Can you work these out from the model? Positions are in its coordinate system, mm. Face numbers are marked on the shaded views. A direction names the side the tool comes from. Give positions to 0.01 mm unless a question says otherwise; leave off trailing zeros. Loops run counter-clockwise (first coordinate to the right, second up) from the corner with the lowest first, then second, coordinate; pieces in that order, holes last.
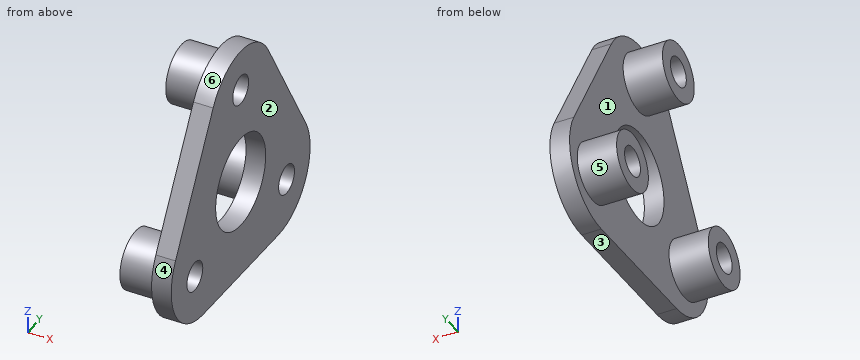
from build123d import *

# Parameters (mm, degrees)
SKETCH_R      = 4.725
SKETCH_R_2    = 1.5
PAD_DEPTH     = 2
SKETCH001_R   = 3
SKETCH001_R_2 = 1.5
PAD001_DEPTH  = 4
FILLET_R      = 6


with BuildPart() as part:
    # Sketch → Pad (new body)
    with BuildSketch(Plane.YZ):
        Polygon((0, 20.207259), (-17.5, -10.10363), (17.5, -10.10363), align=None)
        Circle(SKETCH_R, mode=Mode.SUBTRACT)
        with Locations((0, 10)):
            Circle(SKETCH_R_2, mode=Mode.SUBTRACT)
        with Locations((-8.660254, -5)):
            Circle(SKETCH_R_2, mode=Mode.SUBTRACT)
        with Locations((8.660254, -5)):
            Circle(SKETCH_R_2, mode=Mode.SUBTRACT)
    extrude(amount=-PAD_DEPTH)

    # Sketch001 (on Face9 of Pad) → Pad001 (join)
    with BuildSketch(Plane(origin=(-2, 0, 0), x_dir=(0, 1, 0), z_dir=(-1, 0, 0))):
        with Locations((8.660254, 5)):
            Circle(SKETCH001_R)
        with Locations((8.660254, 5)):
            Circle(SKETCH001_R_2, mode=Mode.SUBTRACT)
        with Locations((-8.660254, 5)):
            Circle(SKETCH001_R)
        with Locations((-8.660254, 5)):
            Circle(SKETCH001_R_2, mode=Mode.SUBTRACT)
        with Locations((0, -10)):
            Circle(SKETCH001_R)
        with Locations((0, -10)):
            Circle(SKETCH001_R_2, mode=Mode.SUBTRACT)
    extrude(amount=PAD001_DEPTH)

    # Fillet
    fillet_edges = [part.edges().sort_by_distance(p)[0] for p in [
        (-1, 0, 20.207259),
        (-1, -17.5, -10.10363),
        (-1, 17.5, -10.10363),
    ]]
    fillet(fillet_edges, radius=FILLET_R)


solid = part.part
(1) Suppose I cut it at C-C on z = 0. List the corners of the cut face in (x, y) for me (3 decimals).
Returned:
outline: (-2, -11.667) - (0, -11.667) - (0, -4.725) - (-2, -4.725) - close; (-2, 4.725) - (0, 4.725) - (0, 11.667) - (-2, 11.667) - close
(2) Please list where these lines run through material, in increasing order: probe 1 along Z at (x, y) = (-0.6, 0) (3 decimals); probe 2 along Y at (x, z) = (-4.2, 10); probe 3 along Y at (x, z) = (-0.4, -5.5).
Returned:
probe 1: z = -10.104 to -4.725, 4.725 to 8.5, 11.5 to 14.207
probe 2: y = -3 to -1.5, 1.5 to 3
probe 3: y = -12.94 to -10.07, -7.25 to 7.25, 10.07 to 12.94
(3) Which directions (+Z, -Z, +X, -X, +Y, -Y) give clear straight access to the entire face, cutting with the end or side of a thin tool? Please do the marked faces 1 and 2.
Returned:
face 1: -X
face 2: +Z, -Z, +X, +Y, -Y
(4) Will these pins go through, and if not, where does the flat tip stop? P1, Ø8, axis at y = 8, z = 3, coming from the +X side; P2, Ø2, axis at x = -1, y = 3.5, coming from the +Z side; P3, Ø1.5, axis at x = -3, y = 3.5, coming from the +Z side; P4, Ø3, axis at x = -2, z = 6, coming from the -Y side.
Returned:
P1: stops at x = 0
P2: stops at z = 13.66
P3: stops at z = 11.2
P4: stops at y = -9.07
(5) Suppose I cut it at A-A on x = -4.2. List the corners of the cut face in (y, z) for me, plus the area to 3 significant figures.
Returned:
outline: circle Ø6 at (-8.66, -5); circle Ø6 at (0, 10); circle Ø6 at (8.66, -5); hole circle Ø3 at (-8.66, -5); hole circle Ø3 at (0, 10); hole circle Ø3 at (8.66, -5)
area: 63.6 mm2
(6) Suppose I cut it at B-B on y = 0. List the corners of the cut face in (x, z) for me (3 decimals), plus the area to 3 significant figures.
Returned:
outline: (-6, 7) - (-2, 7) - (-2, 4.725) - (0, 4.725) - (0, 8.5) - (-6, 8.5) - close; (-6, 11.5) - (0, 11.5) - (0, 14.207) - (-2, 14.207) - (-2, 13) - (-6, 13) - close; (-2, -10.104) - (0, -10.104) - (0, -4.725) - (-2, -4.725) - close
area: 35.7 mm2
(7) Thinking about a two-plate mould opening in Y: for the marked faces 3, 4, 5 and 6, which applies, pulls with the +Y half, pulls with the -Y half, needs draft (parallel to the pull), parting line crosses it, or undercut?
Returned:
face 3: needs draft
face 4: pulls with the -Y half
face 5: undercut
face 6: parting line crosses it
(8) Suppose I cut it at D-D on x = -1.5. List the corners of the cut face in (y, z) for me (3 decimals).
Returned:
outline: (-12.304, -1.104) arc R6 ccw to (-7.108, -10.104) - (7.108, -10.104) arc R6 ccw to (12.304, -1.104) - (5.196, 11.207) arc R6 ccw to (-5.196, 11.207) - close; hole circle Ø3 at (-8.66, -5); hole circle Ø9.45 at (0, 0); hole circle Ø3 at (0, 10); hole circle Ø3 at (8.66, -5)
